Geometry: see drawing. Coordinates: mm, zero at the bounding-box minimum. A direction names the side the tool comes from. Give positions to 0.01 mm unless a question says otherwise; leave off trailing zeros. Loops run counter-clockwise (first coordinate to the right, second up) from the corner with the lowest first, then second, coordinate; pieces in that order, holes last. Notation, with made-up numbers: (-13, -35) -> (18, -35) arc R32 ccw to (18, -3) -> close; hole circle Ø6 at (35, 71.5). An arc over 180 degrees is marked (long way). Return JSON: item names as keys, results as strings. Group by question number.
(1) Cut plane B-B on y = 3. Return loops of the section in (x, z).
(2) Access query for the marked faces 1, 2 and 3. Directions: +Z, -Z, +X, -X, +Y, -Y. A direction counts if a zero-diameter tool reaches every point of the face in a straight line with its end or side. Return the directions, or none.
(3) Ray query, line 1 (Y direction, x = 47, z = 9.5); line 2 (Z direction, x = 3, y = 10.25). Return the intervals inside material, ascending. Write a range as from..to.
(4) Cut plane D-D on x = 3.5. Return loops of the section in (y, z) (1 decimal).
(5) Cut plane C-C on z = 16.5. Return loops of the section in (x, y).
(6) Pin query (flat end, axial travel): pin 1 (1.1 mm diameter, centred on y = 2, z = 16.5, fed in from -X); pin 2 (1.9 mm diameter, centred on x = 3.5, y = 6, fed in from +Z); pin 3 (4 mm diameter, centred on x = 31.5, y = 11, fed in from -Z); pin 4 (7 mm diameter, centred on y = 10, z = 11.5, fed in from +X). Return the tip coordinate at first contact, or that it passes through.
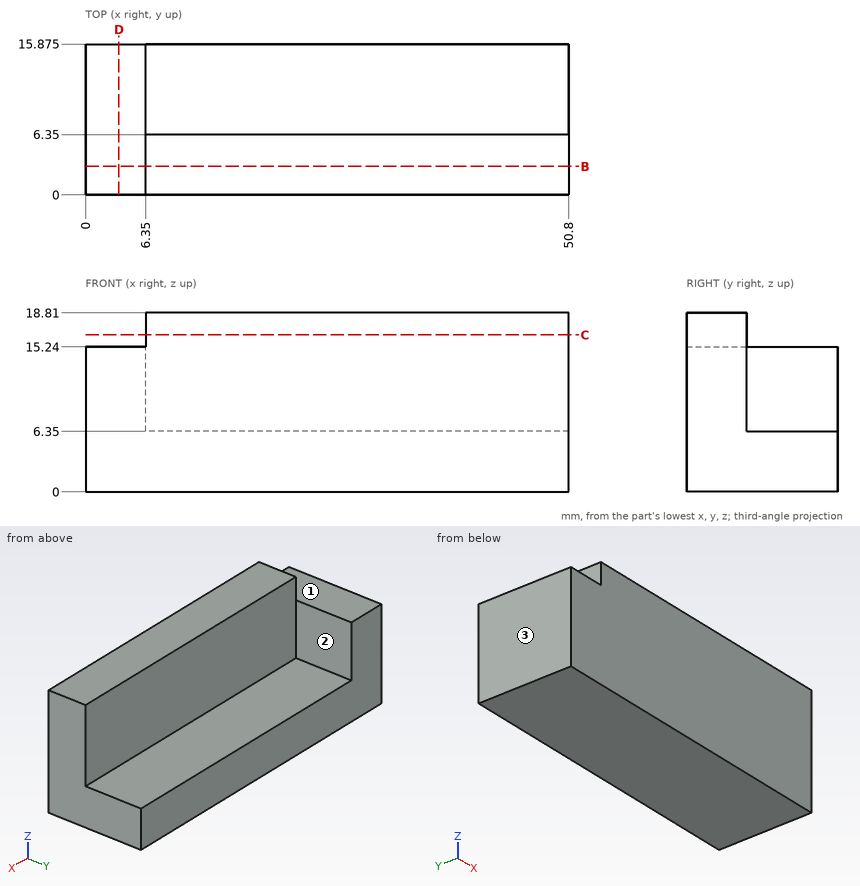
Answers:
{
 "1": {"outline": "(0, 0) -> (50.8, 0) -> (50.8, 18.81) -> (6.35, 18.81) -> (6.35, 15.24) -> (0, 15.24) -> close"},
 "2": {"face 1": "+Z, -X, +Y, -Y", "face 2": "+Z, +X, +Y", "face 3": "+Z, -Z, -X, +Y, -Y"},
 "3": {"line 1": "0..6.35", "line 2": "0..15.24"},
 "4": {"outline": "(0, 0) -> (15.9, 0) -> (15.9, 15.2) -> (0, 15.2) -> close"},
 "5": {"outline": "(6.35, 0) -> (50.8, 0) -> (50.8, 6.35) -> (6.35, 6.35) -> close"},
 "6": {"pin 1": "x = 6.35", "pin 2": "z = 15.24", "pin 3": "z = 0", "pin 4": "x = 6.35"}
}
